Design review of the part built by this model. Coordinates are the model's own, in mm. A direction names the side the tool comes from. Give positions to 0.01 mm unless a question says otherwise; leave off trailing zeros. Order: outer loops, then holes, each group sorted by start corner. A loop starts at its lowest first (then second) coordinate and runs counter-clockwise, first axis right, second up. Notation, with made-up numbers: (33.5, 1.5) -> (86.5, 1.5) arc R4 ccw to (86.5, 5.5) -> close; hole circle Ø8 at (-10.75, 77). An arc over 180 degrees is marked (long way). One line per item, written item: value.
Autodesk Inventor part; units mm, degrees
ref_plane "YZ Plane" through (0, 0, 0) normal (1, 0, 0) x (0, 1, 0)
ref_plane "XZ Plane" through (0, 0, 0) normal (0, 1, 0) x (-1, 0, 0)
ref_plane "XY Plane" through (0, 0, 0) normal (0, 0, 1) x (1, 0, 0)
sketch "Esquisse1" plane through (0, 0, 0) normal (0, 0, 1) x (1, 0, 0)
  line L0 (0, 0) -> (50, 0)
  line L1 (50, 0) -> (50, 55)
  line L2 (50, 55) -> (0, 55)
  line L3 (0, 55) -> (0, 0)
  dimension "d0" = 50
  dimension "d1" = 55
extrude "Extrusion1" add sketch "Esquisse1" along normal blind 1.7
sketch "Esquisse2" plane through (0, 0, 1.7) normal (0, 0, 1) x (1, 0, 0)
  line L0 (0, 0) -> (50, 0) construction
  line L1 (50, 0) -> (50, 55) construction
  line L2 (50, 55) -> (0, 55) construction
  line L3 (0, 55) -> (0, 0) construction
  line L4 (25, 55) -> (25, 0) construction
  line L5 (0, 27.5) -> (50, 27.5) construction
  circle A0 centre (2.8, 52.2) radius 1.5
  line L6 (2.8, 52.2) -> (2.8, 55) construction
  line L7 (2.8, 52.2) -> (0, 52.2) construction
  circle A1 centre (47.2, 52.2) radius 1.5
  circle A2 centre (2.8, 2.8) radius 1.5
  circle A3 centre (47.2, 2.8) radius 1.5
  dimension "d4" = 2.8
  dimension "d5" = 3
extrude "Extrusion2" cut sketch "Esquisse2" against normal blind 1.7
sketch "Esquisse3" plane through (0, 0, 1.7) normal (0, 0, 1) x (1, 0, 0)
  line L0 (50, 0) -> (50, 55) construction
  line L1 (0, 55) -> (0, 0) construction
  line L2 (15, 55) -> (35, 55)
  line L3 (35, 55) -> (35, 0)
  line L4 (35, 0) -> (15, 0)
  line L5 (15, 0) -> (15, 55)
  line L6 (15, 27.5) -> (0, 27.5) construction
  line L7 (35, 27.5) -> (50, 27.5) construction
  dimension "d8" = 20
  dimension "d9" = 55
extrude "Extrusion3" add sketch "Esquisse3" along normal blind 8.5
sketch "Esquisse4" plane through (0, 0, 0) normal (0, -1, 0) x (1, 0, 0)
  line L0 (0, 0) -> (50, 0)
  line L1 (35, 1.7) -> (50, 1.7)
  line L2 (35, 1.7) -> (35, 10.2)
  line L3 (15, 10.2) -> (35, 10.2)
  line L4 (15, 1.7) -> (15, 10.2)
  line L5 (17, 10.2) -> (33, 10.2)
  line L6 (33, 10.2) -> (33, 1.7)
  line L7 (33, 1.7) -> (17, 1.7)
  line L8 (17, 1.7) -> (17, 10.2)
  line L9 (25, 1.7) -> (25, 0) construction
  line L10 (39.3041, 1.7) -> (39.3041, 0) construction
  dimension "d12" = 2
  dimension "d13" = 2
extrude "Extrusion4" cut sketch "Esquisse4" against normal through all
sketch "Esquisse5" plane through (0, 0, 10.2) normal (0, 0, 1) x (1, 0, 0)
  line L0 (33, 55) -> (33, 0) construction
  line L1 (35, 55) -> (33, 55) construction
  line L2 (35, 0) -> (35, 55) construction
  line L3 (33, 0) -> (35, 0) construction
  line L4 (15, 55) -> (35, 55)
  line L5 (35, 55) -> (35, 0)
  line L6 (35, 0) -> (15, 0)
  line L7 (15, 0) -> (15, 55)
  point P0 (0, 0)
extrude "Extrusion5" add sketch "Esquisse5" along normal blind 5
sketch "Esquisse6" plane through (0, 0, 15.2) normal (0, 0, 1) x (1, 0, 0)
  line L0 (35, 55) -> (15, 55) construction
  line L1 (15, 55) -> (15, 0) construction
  line L2 (35, 0) -> (35, 55) construction
  line L3 (21, 55) -> (29, 55)
  line L4 (29, 55) -> (29, 46)
  line L5 (29, 46) -> (21, 46)
  line L6 (21, 46) -> (21, 55)
  line L7 (21, 50.5) -> (15, 50.5) construction
  line L8 (29, 50.5) -> (35, 50.5) construction
  point P0 (0, 0)
  dimension "d18" = 8
  dimension "d19" = 9
extrude "Extrusion6" add sketch "Esquisse6" along normal blind 2.5
sketch "Esquisse7" plane through (0, 0, 0) normal (0, 0, -1) x (-1, 0, 0)
  line L0 (0, 0) -> (-50, 0) construction
  line L1 (0, 55) -> (0, 0) construction
  line L2 (-50, 0) -> (-50, 55) construction
  line L3 (-37, 40) -> (-13, 40)
  line L4 (-13, 40) -> (-13, 12.7126)
  line L5 (-17, 7) -> (-33, 7)
  line L6 (-37, 12.7126) -> (-37, 40)
  line L7 (-37, 23.5) -> (-50, 23.5) construction
  line L8 (-13, 23.5) -> (0, 23.5) construction
  line L9 (-37, 12.7126) -> (-33, 7)
  line L10 (-17, 7) -> (-13, 12.7126)
  dimension "d23" = 7
  dimension "d24" = 24
  dimension "d28" = 145
  dimension "d29" = 145
  dimension "d30" = 33
  dimension "d31" = 4
extrude "Extrusion7" add sketch "Esquisse7" along normal blind 9
sketch "Esquisse8" plane through (0, 0, -9) normal (0, 0, -1) x (-1, 0, 0)
  line L0 (-17, 7) -> (-13, 12.7126) construction
  line L1 (-13, 12.7126) -> (-13, 40) construction
  circle A0 centre (-25.1584, 12.7126) radius 1
  line L2 (-13, 12.7126) -> (-37, 12.7126) construction
  line L3 (-33, 7) -> (-25.1584, 12.7126) construction
  line L4 (-25.1584, 12.7126) -> (-17, 7) construction
  point P0 (0, 0)
  dimension "d32" = 2
extrude "Extrusion8" add sketch "Esquisse8" along normal blind 30
sketch "Esquisse9" plane through (0, 0, 1.7) normal (0, 0, 1) x (1, 0, 0)
  line L0 (50, 0) -> (50, 55) construction
  line L1 (50, 55) -> (35, 55) construction
  line L2 (50, 48) -> (42, 48)
  line L3 (42, 48) -> (42, 13)
  line L4 (42, 13) -> (50, 13)
  line L5 (50, 13) -> (50, 48)
  line L6 (42, 48) -> (42, 55) construction
  point P0 (0, 0)
  dimension "d35" = 0
  dimension "d36" = 8
  dimension "d37" = 35
  dimension "d38" = 7
extrude "Extrusion9" add sketch "Esquisse9" along normal blind 20
equation "\"d13\" = d12"
equation "\"d29\" = d28"
properties part number "CarteElectronique"
Item 1: Clearance check with flat-ended pins moving along their axes: P1, Ø10, axis at x = 20.5, y = 6, coming from the -Z side; P2, Ø2, axis at y = 51, z = 16.5, coming from the +X side; P3, Ø3.5, axis at x = 2.8, y = 2.8, coming from the +Z side; P4, Ø1.5, axis at y = 26, z = -0.5, coming from the -X side. State where each tip first meets the part, or that it passes through.
Returned:
P1: z = -9
P2: x = 29
P3: z = 1.7
P4: x = 0
Item 2: Add section B-B on z = 13. Give the boundary of the cut face in (x, y), plus the area to 3 significant figures.
Returned:
outline: (15, 0) -> (35, 0) -> (35, 55) -> (15, 55) -> close; (42, 13) -> (50, 13) -> (50, 48) -> (42, 48) -> close
area: 1,380 mm²
Item 3: Machinability: for faces 1 (the flat face through (13, 27, -4)), 2 (the flat face through (15, 27, 8)), 3 (the flat face through (25, 40, -4)), 4 (the flat face through (29, 51, 16)), 5 (the flat face through (25, 46, 16)), which of the approach directions +Z, -Z, +X, -X, +Y, -Y give a long, thin tool a straight path to every point of the face, cutting with its end or side? Answer none if there is none.
Returned:
face 1: -Z, -X, +Y, -Y
face 2: +Z, -X, +Y, -Y
face 3: -Z, +X, -X, +Y
face 4: +Z, +Y, -Y
face 5: +Z, -X, -Y
Item 4: Add section C-C on x = 47.2. Give the boundary of the cut face in (y, z), plus the area to 3 significant figures.
Returned:
outline: (0, 0) -> (1.3, 0) -> (1.3, 1.7) -> (0, 1.7) -> close; (4.3, 0) -> (50.7, 0) -> (50.7, 1.7) -> (48, 1.7) -> (48, 21.7) -> (13, 21.7) -> (13, 1.7) -> (4.3, 1.7) -> close; (53.7, 0) -> (55, 0) -> (55, 1.7) -> (53.7, 1.7) -> close
area: 783 mm²
Item 5: Add section A-A on y = 52.2. Give the boundary of the cut face in (x, z).
Returned:
outline: (0, 0) -> (1.3, 0) -> (1.3, 1.7) -> (0, 1.7) -> close; (4.3, 0) -> (45.7, 0) -> (45.7, 1.7) -> (35, 1.7) -> (35, 15.2) -> (29, 15.2) -> (29, 17.7) -> (21, 17.7) -> (21, 15.2) -> (15, 15.2) -> (15, 1.7) -> (4.3, 1.7) -> close; (48.7, 0) -> (50, 0) -> (50, 1.7) -> (48.7, 1.7) -> close; hole (17, 1.7) -> (33, 1.7) -> (33, 10.2) -> (17, 10.2) -> close
Item 6: To check wall thickness, follow line 1 along Y through (x, z) = (47.2, 0.9); line 2 along X through (y, z) = (38.5, 7); line 3 along X through (y, z) = (52, 1). State the ranges of each line that lie inside material, in increasing order. Write a range as from..to.
Returned:
line 1: 0..1.3, 4.3..50.7, 53.7..55
line 2: 15..17, 33..35, 42..50
line 3: 0..1.31, 4.29..45.71, 48.69..50
Item 7: Draft analysis for pull direction X (two halves, no side actions). For faces 6 (the flat face through (21, 50, 16)), 7 (the flat face through (25, 7, -4)), 8 (the flat face through (17, 27, 6)), state which applies: pulls with the +X half, pulls with the -X half, needs draft (parallel to the pull), parting line crosses it, or undercut.
Returned:
face 6: pulls with the -X half
face 7: needs draft
face 8: undercut
Item 8: Add section D-D on y = 2.8. Give the boundary of the cut face in (x, z).
Returned:
outline: (0, 0) -> (1.3, 0) -> (1.3, 1.7) -> (0, 1.7) -> close; (4.3, 0) -> (45.7, 0) -> (45.7, 1.7) -> (35, 1.7) -> (35, 15.2) -> (15, 15.2) -> (15, 1.7) -> (4.3, 1.7) -> close; (48.7, 0) -> (50, 0) -> (50, 1.7) -> (48.7, 1.7) -> close; hole (17, 1.7) -> (33, 1.7) -> (33, 10.2) -> (17, 10.2) -> close
